Work out the finished part from the listing and answer in its coordinate system (mm). A direction names the side the tool comes from. Give positions to 0.01 mm unless a question says otherwise; leave off trailing zeros. Order: outer loops, then holes, each group sorted by start corner. A loop starts at its lowest first (then second) coordinate and runs counter-clockwise, first axis right, second up.
```python
from build123d import *

# Parameters (mm, degrees)
SKETCH1_W           = 762
SKETCH1_H           = 228.6
BOSS_EXTRUDE1_DEPTH = 76.2
SKETCH2_W           = 203.2
SKETCH2_H           = 95.25
CUT_EXTRUDE1_DEPTH  = 63.5
SKETCH3_W           = 203.2
SKETCH3_H           = 50.8
CUT_EXTRUDE2_DEPTH  = 799.081581043
FILLET1_R           = 25.4
SKETCH4_R           = 1.016
CUT_EXTRUDE3_DEPTH  = 800.192342306
LPATTERN1_COUNT     = 4
LPATTERN1_PITCH     = 152.4
FILLET2_R           = 6.35
FILLET3_R           = 6.35
SKETCH6_R           = 1.016
CUT_EXTRUDE4_DEPTH  = 50.8


with BuildPart() as part:
    # Sketch1 → Boss-Extrude1 (new body)
    with BuildSketch(Plane(origin=(0, 0, 0), x_dir=(0, 0, -1), z_dir=(1, 0, 0))):
        with Locations((381, 114.3)):
            Rectangle(SKETCH1_W, SKETCH1_H)
    extrude(amount=BOSS_EXTRUDE1_DEPTH)

    # Sketch2 → Cut-Extrude1 (cut)
    with BuildSketch(Plane.ZY):
        with Locations((-381, 92.075)):
            Rectangle(SKETCH2_W, SKETCH2_H)
    extrude(amount=-CUT_EXTRUDE1_DEPTH, mode=Mode.SUBTRACT)

    # Sketch3 → Cut-Extrude2 (cut, through all)
    with BuildSketch(Plane.ZY.offset(-63.5)):
        with Locations((-381, 82.55)):
            Rectangle(SKETCH3_W, SKETCH3_H)
    extrude(amount=-CUT_EXTRUDE2_DEPTH, mode=Mode.SUBTRACT)

    # Fillet1
    fillet1_edges = [part.edges().sort_by_distance(p)[0] for p in [
        (31.75, 139.7, -482.6),
        (31.75, 139.7, -279.4),
    ]]
    fillet(fillet1_edges, radius=FILLET1_R)

    # Sketch4 → Cut-Extrude3 (cut, through all)
    with BuildSketch(Plane.ZY):
        with Locations((-609.6, 25.4)):
            Circle(SKETCH4_R)
    cut_extrude3 = extrude(amount=-CUT_EXTRUDE3_DEPTH, mode=Mode.SUBTRACT)

    # LPattern1: Cut-Extrude3 ×4
    with Locations(*[(0, 0, i * LPATTERN1_PITCH) for i in range(1, LPATTERN1_COUNT)]):
        add(cut_extrude3, mode=Mode.SUBTRACT)

    # Fillet2
    fillet2_edges = [part.edges().sort_by_distance(p)[0] for p in [
        (69.85, 57.15, -482.6),
        (69.85, 107.95, -482.6),
        (69.85, 107.95, -279.4),
        (69.85, 57.15, -279.4),
    ]]
    fillet(fillet2_edges, radius=FILLET2_R)

    # Fillet3
    fillet3_edges = [part.edges().sort_by_distance(p)[0] for p in [
        (31.75, 44.45, -482.6),
        (31.75, 44.45, -279.4),
    ]]
    fillet(fillet3_edges, radius=FILLET3_R)

    # Sketch6 → Cut-Extrude4 (cut)
    with BuildSketch(Plane(origin=(0, 228.6, 0), x_dir=(1, 0, 0), z_dir=(0, 1, 0))):
        with Locations(Location((38.1, 571.5, 0), (0, 0, 270))):
            Circle(SKETCH6_R)
        with Locations(Location((38.1, 190.5, 0), (0, 0, 270))):
            Circle(SKETCH6_R)
    extrude(amount=-CUT_EXTRUDE4_DEPTH, mode=Mode.SUBTRACT)


solid = part.part
```
1. Which of the six approach directions +Z, -Z, +X, -X, +Y, -Y give full straight-line access (tool end or side, diameter ignored) to faces 1 (the face through (63.5, 121, -382)), 2 (the face through (38, 113, 0)), 3 (the face through (70, 57.15, -382))?
Findings below:
face 1: -X
face 2: +Z, +X, -X, +Y, -Y
face 3: +X, -X
2. Given P1, Ø5.5, axis at y = 57, z = -356.5, coming from the -X side; P2, Ø3.5, axis at y = 25.4, z = -152.4, coming from the -X side; P3, Ø1.2, axis at y = 25.4, z = -457.2, coming from the -X side, each flat-ended and moving along its own axis, determine where each tip first touches the part or whether it passes through.
Findings below:
P1: stops at x = 63.5
P2: stops at x = 0
P3: passes through
3. The mould has two halves that part along Y. Classify faces 4 (the face through (0, 141, -376)), 5 (the face through (38, 0, -376)), 6 (the face through (70, 107.95, -382)): pulls with the +Y half, pulls with the -Y half, needs draft (parallel to the pull), parting line crosses it, or undercut.
Findings below:
face 4: needs draft
face 5: pulls with the -Y half
face 6: undercut
4. Straight lines are drawn through the part: probe 1 along Z at (x, y) = (38, 192); probe 2 along Z at (x, y) = (44, 25); probe 3 along X at (y, z) = (203, -571.5). For each, find the intervals that lie inside material, in ascending order.
Findings below:
probe 1: z = -762 to -572.51, -570.49 to -191.51, -189.49 to 0
probe 2: z = -762 to -610.53, -608.67 to -458.13, -456.27 to -305.73, -303.87 to -153.33, -151.47 to 0
probe 3: x = 0 to 37.08, 39.12 to 76.2
5. The part is cut by section A-A (x = 18). Write down the section's boundary in (y, z), then the cut area to 3 significant figures.
Findings below:
outline: (0, -762) - (228.6, -762) - (228.6, 0) - (0, 0) - close; hole circle Ø2.03 at (25.4, -609.6); hole circle Ø2.03 at (25.4, -457.2); hole circle Ø2.03 at (25.4, -304.8); hole circle Ø2.03 at (25.4, -152.4); hole (44.45, -476.25) arc R6.35 ccw to (50.8, -482.6) - (114.3, -482.6) arc R25.4 ccw to (139.7, -457.2) - (139.7, -304.8) arc R25.4 ccw to (114.3, -279.4) - (50.8, -279.4) arc R6.35 ccw to (44.45, -285.75) - close
area: 155,000 mm2
